```python
from build123d import *

# Parameters (mm, degrees)
EXTRUDE_1_DEPTH     = 30
SKETCH_2_R          = 7.5
CUT_EXTRUDE_1_DEPTH = 71.356236397
SKETCH_5_R          = 2.6
CUT_EXTRUDE_4_DEPTH = 80.376381878
SKETCH_6_R          = 2.6
CUT_EXTRUDE_5_DEPTH = 80.376381878


with BuildPart() as part:
    # 草图1 → 凸台-拉伸1 (new body)
    with BuildSketch(Plane.XY):
        Polygon((-15, -15), (-13.1, -15), (-13.1, -45), (-10.1, -45), (-10.1, -15), (10.1, -15), (10.1, -45), (13.1, -45), (13.1, -15), (15, -15), (15, 15), (-15, 15), (-15, 13.1), (-45, 13.1), (-45, 10.1), (-15, 10.1), (-15, -10.1), (-45, -10.1), (-45, -13.1), (-15, -13.1), align=None)
    extrude(amount=EXTRUDE_1_DEPTH)

    # 草图2 → 切除-拉伸1 (cut, through all)
    with BuildSketch(Plane.XY.offset(30)):
        Circle(SKETCH_2_R)
    extrude(amount=-CUT_EXTRUDE_1_DEPTH, mode=Mode.SUBTRACT)

    # 草图5 → 切除-拉伸4 (cut, through all)
    with BuildSketch(Plane(origin=(13.1, 0, 0), x_dir=(0, 0, -1), z_dir=(1, 0, 0))):
        with Locations(Location((-15, -23, 0), (0, 0, 90))):
            Circle(SKETCH_5_R)
        with Locations(Location((-15, -36, 0), (0, 0, 90))):
            Circle(SKETCH_5_R)
    extrude(amount=-CUT_EXTRUDE_4_DEPTH, mode=Mode.SUBTRACT)

    # 草图6 → 切除-拉伸5 (cut, through all)
    with BuildSketch(Plane(origin=(0, 13.1, 0), x_dir=(1, 0, 0), z_dir=(0, 1, 0))):
        with Locations(Location((-23, -15, 0), (0, 0, 180))):
            Circle(SKETCH_6_R)
        with Locations(Location((-36, -15, 0), (0, 0, 180))):
            Circle(SKETCH_6_R)
    extrude(amount=-CUT_EXTRUDE_5_DEPTH, mode=Mode.SUBTRACT)


solid = part.part
```
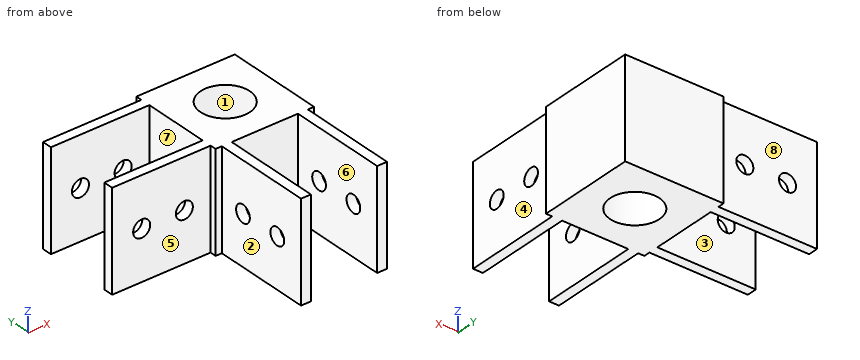
Here's how the part is built. I have some questions about the finished solid (model axes, mm). Face numbers are marked on the shaded views. A direction names the side the tool comes from. Give positions to 0.01 mm unless a question says otherwise; leave off trailing zeros. Loops run counter-clockwise (first coordinate to the right, second up) from the corner with the lowest first, then second, coordinate; pieces in that order, holes last. Notation, with made-up numbers: M 54.25,28 L 108.25,28 A26 cw 108.25,44 Z; hole C 16,52.25 d5. An arc over 180 degrees is marked long. Return JSON: item names as keys, results as strings.
Item 1: Imagine slicing it at A-A on y = -31.5. List the corners of the cut face in (x, z) for me.
A:
{"outline": "M -13.1,0 L -10.1,0 L -10.1,30 L -13.1,30 Z; M 10.1,0 L 13.1,0 L 13.1,30 L 10.1,30 Z"}
Item 2: Thinking about a two-plate mould opening in X: for the marked faces 1, 2, 3 and 4, which applies, released by +X, released by -X, zero draft, split by the parting line, or undercut?
A:
{"face 1": "undercut", "face 2": "released by -X", "face 3": "zero draft", "face 4": "released by +X"}
Item 3: On a 3-axis mill with a long thin cutter (end or side, diameter ignored), from which of +Z, -Z, +X, -X, +Y, -Y can I reach the whole of each face in a straight line? I mean the marked faces 5, 6, 7 and 8. Say none if no direction works.
A:
{"face 5": "+Z, -Z, -X, -Y", "face 6": "+Z, -Z, -Y", "face 7": "+Z, -Z, -X", "face 8": "+Z, -Z, -X, +Y"}
Item 4: Imagine slicing it at C-C on z = 7.75. List the corners of the cut face in (x, y) for me, then the cut area to 3 significant figures.
A:
{"outline": "M -45,-13.1 L -15,-13.1 L -15,-15 L -13.1,-15 L -13.1,-45 L -10.1,-45 L -10.1,-15 L 10.1,-15 L 10.1,-45 L 13.1,-45 L 13.1,-15 L 15,-15 L 15,15 L -15,15 L -15,13.1 L -45,13.1 L -45,10.1 L -15,10.1 L -15,-10.1 L -45,-10.1 Z; hole C 0,0 d15", "area": "1,080 mm^2"}
Item 5: Please list where these lines run through material, in increasing order: line 1 (X direction, y = -30.5, z = 24.5); line 2 (Y direction, x = 0, z = 7.25).
A:
{"line 1": "x = -13.1 to -10.1, 10.1 to 13.1", "line 2": "y = -15 to -7.5, 7.5 to 15"}
Item 6: Imagine slicing it at D-D on x = -36. List the corners of the cut face in (y, z) for me, then the cut area to 3 significant figures.
A:
{"outline": "M -13.1,0 L -10.1,0 L -10.1,12.4 L -13.1,12.4 Z; M -13.1,17.6 L -10.1,17.6 L -10.1,30 L -13.1,30 Z; M 10.1,0 L 13.1,0 L 13.1,12.4 L 10.1,12.4 Z; M 10.1,17.6 L 13.1,17.6 L 13.1,30 L 10.1,30 Z", "area": "149 mm^2"}
Item 7: I'm going to push flat-ended pins straight in: pin 1 Ø6 at (y, z) = (-36, 15) entering from -X; pin 2 Ø6 at (y, z) = (-2, 19.5) entering from -X; pin 3 Ø6 at (x, z) = (-8, 11.5) entering from -Y; pin 4 Ø4 at (y, z) = (-36, 15) entering from +X. Where does each tip first touch, or does it pass through?
A:
{"pin 1": "stops at x = -13.1", "pin 2": "stops at x = -15", "pin 3": "stops at y = -45", "pin 4": "passes through"}
